Read the model definition and answer for the solid it produces. Units are mm, in the model's axes. A direction names the side the tool comes from. Give positions to 0.01 mm unless a question says otherwise; leave off trailing zeros. Order: outer loops, then holes, each group sorted by start corner. A loop starts at its lowest first (then second) coordinate and runs counter-clockwise, first axis right, second up.
Item 1: Given pin 1 Ø4 at (x, y) = (-31.5, -15.5) entering from -Z; pin 2 Ø10 at (y, z) = (-15.5, 7) entering from -X; pin 3 Ø8 at (x, y) = (-14, -6.5) entering from +Z, each flat-ended and moving along its own axis, determine where each tip first touches the part or whether it passes through.
Item 2: Which of the six approach directions +Z, -Z, +X, -X, +Y, -Y give full straight-line access (tool end or side, diameter ignored) to faces 4 (the face through (-1, -13, -6.35)), 5 (the face through (-25, -13, 12.7)), 6 (the face through (0, -13, 6.35))?
Item 3: A cutting plane is placed at A-A (y = -2.5). Write down the section's boundary in (x, z).
Item 4: The mould has two halves that part along Z. Classify faces 1 (the face through (-17.85, -12.52, 10.95)), 2 (the face through (-14, 0, 0)), 3 (the face through (-16.294, -12.522, 3.052)): +Z half, -Z half, draft (parallel to the pull), parting line (faces both ways), or undercut.
Item 5: Find the intervals of material crossed by line 1 along Z through (x, y) = (-26, -17.5); line 2 along Z through (x, y) = (-2.5, -18.25); line 3 along X through (y, z) = (-8.5, -0.5), in increasing order.
Item 6: A cutting plane is placed at D-D (z = 7). Write down the section's boundary in (x, y), plus the area to 3 significant figures.
Item 7: A cutting plane is placed at B-B (z = 1). Write down the section's boundary in (x, y).
Item 8: A cutting plane is placed at C-C (x = -7). Write down the section's boundary in (y, z), plus the area to 3 significant figures.
from build123d import *

# Parameters (mm, degrees)
F0_R        = 10.16
F1_DEPTH    = 25.4
F2_T1_DEPTH = 80.3926131403
F2_T3_DEPTH = 88.9


# Not quite as in the source:
# - a fillet or chamfer that OpenCascade refuses, or shapes differently, is made with other operations: its cross-section is extruded or revolved along the edge and cut away or added


with BuildPart() as f1:
    # F0 (on Front) → F1 (new body)
    with BuildSketch(Plane.XZ):
        Polygon((-13.2853005409, 12.7), (-38.6853005409, 12.7), (-38.6853005409, -12.7), (-13.2853005409, -12.7), (-13.2853005409, -6.35), (12.1146994591, -6.35), (12.1146994591, 6.35), (-13.2853005409, 6.35), align=None)
        with Locations((-25.9853005409, 0)):
            Circle(F0_R, mode=Mode.SUBTRACT)
    extrude(amount=F1_DEPTH)

    # F2: fillet of radius 12.7 on 4 edges, made by hand

    # F2_s2 → F2_t1 (cut)
    with BuildSketch(Plane.XZ.offset(-27.4963065702)):
        with BuildLine():
            ThreePointArc((-13.2853005409, 6.35), (-17.933823169, 10.9985226281), (-24.283823169, 12.7))
            Line((-24.283823169, 12.7), (-13.2853005409, 12.7))
            Line((-13.2853005409, 12.7), (-13.2853005409, 6.35))
        make_face()
        with BuildLine():
            ThreePointArc((-24.283823169, -12.7), (-17.933823169, -10.9985226281), (-13.2853005409, -6.35))
            Line((-13.2853005409, -6.35), (-13.2853005409, -12.7))
            Line((-13.2853005409, -12.7), (-24.283823169, -12.7))
        make_face()
    extrude(amount=F2_T1_DEPTH, mode=Mode.SUBTRACT)

    # F2_s4 → F2_t3 (cut)
    with BuildSketch(Plane.XZ.offset(-31.75)):
        with BuildLine():
            ThreePointArc((-25.9853005409, 12.7), (-34.965556662, 8.9802561211), (-38.6853005409, 0))
            Line((-38.6853005409, 0), (-38.6853005409, 12.7))
            Line((-38.6853005409, 12.7), (-25.9853005409, 12.7))
        make_face()
        with BuildLine():
            ThreePointArc((-38.6853005409, 0), (-34.965556662, -8.9802561211), (-25.9853005409, -12.7))
            Line((-25.9853005409, -12.7), (-38.6853005409, -12.7))
            Line((-38.6853005409, -12.7), (-38.6853005409, 0))
        make_face()
    extrude(amount=F2_T3_DEPTH, mode=Mode.SUBTRACT)


solid = f1.part
Response values:
1. pin 1: stops at z = -12.2
1. pin 2: stops at x = -38.53
1. pin 3: stops at z = 11.04
2. face 4: -Z, +X, +Y, -Y
2. face 5: +Z, +X, -X, +Y, -Y
2. face 6: +Z, +X, +Y, -Y
3. outline: (-25.99, -12.7) - (-24.28, -12.7) arc R12.7 ccw to (-13.29, -6.35) - (12.11, -6.35) - (12.11, 6.35) - (-13.29, 6.35) arc R12.7 ccw to (-24.28, 12.7) - (-25.99, 12.7) arc R12.7 ccw to start; hole circle Ø20.32 at (-25.99, 0)
4. face 1: +Z half
4. face 2: draft
4. face 3: undercut
5. line 1: z = -12.7 to -10.16, 10.16 to 12.7
5. line 2: z = -6.35 to 6.35
5. line 3: x = -38.68 to -36.13, -15.84 to 12.11
6. outline: (-36.58, -25.4) - (-33.35, -25.4) - (-33.35, 0) - (-36.58, 0) - close; (-18.62, -25.4) - (-13.69, -25.4) - (-13.69, 0) - (-18.62, 0) - close
6. area: 207 mm2
7. outline: (-38.65, -25.4) - (-36.1, -25.4) - (-36.1, 0) - (-38.65, 0) - close; (-15.87, -25.4) - (12.11, -25.4) - (12.11, 0) - (-15.87, 0) - close
8. outline: (-25.4, -6.35) - (0, -6.35) - (0, 6.35) - (-25.4, 6.35) - close
8. area: 323 mm2
